Could you check a few things on this model? Use its own coordinates, in mm. Round coordinates to 2 decimals unless told otherwise and drop trailing zeros. Loops run counter-clockwise (first coordinate to the right, second up) from the corner with the lowest first, then second, coordinate; pieces in that order, holes last.
from build123d import *

# Parameters (mm, degrees)
SKETCH1_R          = 9.525
EXTRUDE1_DEPTH     = 59
SKETCH2_R          = 2.38125
SKETCH3_W          = 35.382303839
SKETCH3_H          = 29.228859692
CUT_EXTRUDE1_DEPTH = 10


with BuildPart() as part:
    # Sketch1 → Extrude1 (new body)
    with BuildSketch(Plane.XY):
        Polygon((-12.7, 7.332348419), (-12.7, -7.332348419), (0, -14.664696837), (12.7, -7.332348419), (12.7, 7.332348419), (0, 14.664696837), align=None)
        Circle(SKETCH1_R, mode=Mode.SUBTRACT)
    extrude(amount=-EXTRUDE1_DEPTH)

    # Sketch2 → Cut-Revolve3 (revolve, cut)
    with BuildSketch(Plane(origin=(0, 0, 0), x_dir=(0, 0, -1), z_dir=(1, 0, 0)), mode=Mode.PRIVATE) as cut_revolve3_sk:
        Polygon((59, 14.664696837), (48.285996634, 14.664696837), (49, 12), (59, 12), align=None)
        Polygon((1.964696837, 14.664696837), (0, 14.664696837), (0, 12.7), align=None)
        with Locations((26.9875, 14.78125)):
            Circle(SKETCH2_R)
    revolve(cut_revolve3_sk.sketch.rotate(Axis((0, 0, 0), (0, 0, -1)), 90), axis=Axis((0, 0, 0), (0, 0, -1)), mode=Mode.SUBTRACT)

    # Sketch3 → Cut-Extrude1 (cut)
    with BuildSketch(Plane(origin=(0, 0, -59), x_dir=(-1, 0, 0), z_dir=(0, 0, -1))):
        with Locations((2.307541554, -0.133770525)):
            Rectangle(SKETCH3_W, SKETCH3_H)
    extrude(amount=-CUT_EXTRUDE1_DEPTH, mode=Mode.SUBTRACT)


solid = part.part
Item 1: Will these pins go through, and if not, where does the flat tip stop? pin 1 (6 mm diameter, centred on x = 9.5, z = -39.5, fed in from +Y); pin 2 (2 mm diameter, centred on y = 8.5, z = -29, fed in from -X).
Results list:
pin 1: stops at y = 10.91
pin 2: stops at x = -12.3
Item 2: If I drill on line 1 along Y through (x, z) = (0, -38) (3 decimals); line 2 along X through (y, z) = (3.5, -7); line 3 along Y through (x, z) = (-2, -5), over which ranges is the centre line in solid material (lowest first)?
Results list:
line 1: y = -14.665 to -9.525, 9.525 to 14.665
line 2: x = -12.7 to -8.86, 8.86 to 12.7
line 3: y = -13.51 to -9.31, 9.31 to 13.51
Item 3: If we section it at A-A, the plane z = -16: Please give me the cut outline in (x, y) (3 decimals).
Results list:
outline: (-12.7, -7.332) - (0, -14.665) - (12.7, -7.332) - (12.7, 7.332) - (0, 14.665) - (-12.7, 7.332) - close; hole circle Ø19.05 at (0, 0)
